```python
from build123d import *

# Parameters (mm, degrees)
F1_DEPTH = 4
F2_W     = 4
F2_H     = 12
F3_DEPTH = 22
F5_DEPTH = 25
F7_DEPTH = 1.5
F8_R     = 5


# Not quite as in the source:
# - a feature names something its author has since deleted; it is built from what else it names


with BuildPart() as f1:
    # F0 (on Top) → F1 (new body)
    with BuildSketch(Plane.XY):
        with BuildLine():
            ThreePointArc((0, -3), (-0.8786796564, -0.8786796564), (-3, 0))
            Line((-3, 0), (-40, 0))
            Line((-40, 0), (-40, -12))
            Line((-40, -12), (-3, -12))
            ThreePointArc((-3, -12), (-0.8786796564, -11.1213203436), (0, -9))
            Line((0, -9), (0, -3))
        make_face()
        with BuildLine():
            ThreePointArc((-3, -3.95), (-0.95, -6), (-3, -8.05))
            Line((-3, -8.05), (-14, -8.05))
            ThreePointArc((-14, -8.05), (-16.05, -6), (-14, -3.95))
            Line((-14, -3.95), (-3, -3.95))
        make_face(mode=Mode.SUBTRACT)
    extrude(amount=F1_DEPTH)

    # F2 (on face) → F3 (join)
    with BuildSketch(Plane.XY.offset(4)):
        with Locations((-38, -6)):
            Rectangle(F2_W, F2_H)
    extrude(amount=F3_DEPTH)

    # F4 (on face) → F5 (cut)
    with BuildSketch(Plane(origin=(-40, 0, 0), x_dir=(0, -1, 0), z_dir=(-1, 0, 0))):
        with BuildLine():
            Line((4, 21), (4, 9))
            ThreePointArc((4, 9), (4.5857864376, 7.5857864376), (6, 7))
            ThreePointArc((6, 7), (7.4142135624, 7.5857864376), (8, 9))
            Line((8, 9), (8, 21))
            ThreePointArc((8, 21), (7.4142135624, 22.4142135624), (6, 23))
            ThreePointArc((6, 23), (4.5857864376, 22.4142135624), (4, 21))
        make_face()
    extrude(amount=-F5_DEPTH, mode=Mode.SUBTRACT)

    # F6 (on face) → F7 (cut)
    with BuildSketch(Plane.YZ.offset(-36)):
        Polygon((-6, 4.8430780618), (-2.4, 6.9215390309), (-2.4, 23.0784609691), (-6, 25.1569219382), (-9.6, 23.0784609691), (-9.6, 6.9215390309), align=None)
        with BuildLine():
            ThreePointArc((-8, 21), (-6, 23), (-4, 21))
            Line((-4, 21), (-4, 9))
            ThreePointArc((-4, 9), (-6, 7), (-8, 9))
            Line((-8, 9), (-8, 21))
        make_face(mode=Mode.SUBTRACT)
    extrude(amount=-F7_DEPTH, mode=Mode.SUBTRACT)

    # F8
    f8_edges = [f1.edges().sort_by_distance(p)[0] for p in [
        (-38, -12, 26),
        (-38, 0, 26),
    ]]
    fillet(f8_edges, radius=F8_R)


solid = f1.part
```
Model file for the job. Use its own axes, mm. A direction names the side the tool comes from. Coordinates: 2 decimals unless noted, no trailing zeros. Write each loop counter-clockwise with the first axis right and the second up, starting at its lowest first coordinate (ties: lowest second). Pieces come first, ordered by that corner, then holes. Notation, with made-up numbers: (18, 8) - (62, 8) arc R20 cw to (62, 19) - close; hole circle Ø8 at (-5, 69.5). An arc over 180 degrees is marked (long way). Use a Markdown table: item, result. Add a question column.
Item 1: Drop flat-ended pins along their axis: pin 1 (6 mm diameter, centred on y = -8, z = 10.5, fed in from +X); pin 2 (3.5 mm diameter, centred on y = -5.5, z = 11.5, fed in from +X); pin 3 (1.5 mm diameter, centred on x = -13, y = -4.5, fed in from +Z). Give the stop position or say it passes through.
Item 2: Two-plate mould, pull along Z, no slides. Class faces 1 (the face through (-37.5, -8.5, 15.1)), 2 (the face through (-20, -6, 0)), 3 (the face through (0, -6, 2)), 4 (the face through (-38, -10, 25)): pulls with the +Z half, pulls with the -Z half, needs draft (parallel to the pull), parting line crosses it, or undercut.
Item 3: Band-saw the part on C-C, the plane z = 16. Write the cut outline in (x, y), and give its area (3 significant figures).
Item 4: Band-saw the part on D-D, the plane y = -1. Write the cut outline in (x, z).
Item 5: 3-axis set-ups, long thin cutter, end or side, ignore diameter. For faces 5 (the face through (-39, -4, 15)), 6 (the face through (-9, -3.95, 2)), 7 (the face through (-37, -8, 24)): which of +Z, -Z, +X, -X, +Y, -Y reach the whole face in a straight line?
Item 6: Band-saw the part on B-B, the plane x = -4. Write the cut outline in (y, z), and give its area (3 significant figures).
Item 7: Drill centre lines: line 1 along Z through (x, y) = (-1.5, -2.75); line 2 along X through (y, z) = (-8.25, 10.75); line 3 along X through (y, z) = (-10.5, 12). Where is each one in solid material? Low to high.
Item 8: Band-saw the part on A-A, the plane x = -37. Write the cut outline in (y, z).
A:
| question | item | result |
|---|---|---|
| 1 | pin 1 | stops at x = -36 |
| 1 | pin 2 | stops at x = -37.5 |
| 1 | pin 3 | stops at z = 4 |
| 2 | face 1 | undercut |
| 2 | face 2 | pulls with the -Z half |
| 2 | face 3 | needs draft |
| 2 | face 4 | pulls with the +Z half |
| 3 | outline | (-40, -12) - (-36, -12) - (-36, -9.6) - (-37.5, -9.6) - (-37.5, -8) - (-40, -8) - close; (-40, -4) - (-37.5, -4) - (-37.5, -2.4) - (-36, -2.4) - (-36, 0) - (-40, 0) - close |
| 3 | area | 27.2 mm² |
| 4 | outline | (-40, 0) - (-0.76, 0) - (-0.76, 4) - (-36, 4) - (-36, 24) - (-40, 24) - close |
| 5 | face 5 | +X, -X |
| 5 | face 6 | +Z, -Z |
| 5 | face 7 | +X |
| 6 | outline | (-12, 0) - (-8.05, 0) - (-8.05, 4) - (-12, 4) - close; (-3.95, 0) - (0, 0) - (0, 4) - (-3.95, 4) - close |
| 6 | area | 31.6 mm² |
| 7 | line 1 | z = 0 to 4 |
| 7 | line 2 | x = -40 to -37.5 |
| 7 | line 3 | x = -40 to -36 |
| 8 | outline | (-12, 0) - (0, 0) - (0, 21) arc R5 ccw to (-5, 26) - (-7, 26) arc R5 ccw to (-12, 21) - close; hole (-9.6, 6.92) - (-6, 4.84) - (-2.4, 6.92) - (-2.4, 23.08) - (-6, 25.16) - (-9.6, 23.08) - close |
